from build123d import *

# Parameters (mm, degrees)
F1_W     = 100
F1_H     = 50
F2_DEPTH = 15
F3_R     = 10
F4_R     = 10
F5_W     = 40
F5_H     = 5
F6_DEPTH = 50.001
F7_T     = -3


with BuildPart() as f2:
    # F1 (on Front) → F2 (new body)
    with BuildSketch(Plane.XZ):
        with Locations((50, 25)):
            Rectangle(F1_W, F1_H)
    extrude(amount=F2_DEPTH)

    # F3
    f3_edges = [f2.edges().sort_by_distance(p)[0] for p in [
        (100, -7.5, 50),
    ]]
    fillet(f3_edges, radius=F3_R)

    # F4
    f4_edges = [f2.edges().sort_by_distance(p)[0] for p in [
        (100, -7.5, 0),
    ]]
    fillet(f4_edges, radius=F4_R)

    # F5 (on face) → F6 (cut, through all)
    with BuildSketch(Plane(origin=(0, 0, 0), x_dir=(1, 0, 0), z_dir=(0, 0, -1))):
        with Locations((50, 12.5)):
            Rectangle(F5_W, F5_H)
    extrude(amount=-F6_DEPTH, mode=Mode.SUBTRACT)

    # F7
    f7_openings = [f2.faces().sort_by_distance(p)[0] for p in [
        (49.58642, 0, 25),
    ]]
    offset(amount=F7_T, openings=f7_openings, kind=Kind.INTERSECTION)


solid = f2.part
Here's how the part is built. I have some questions about the finished solid (model axes, mm). A direction names the side the tool comes from. Round coordinates to 2 decimals unless told otherwise and drop trailing zeros. Loops run counter-clockwise (first coordinate to the right, second up) from the corner with the lowest first, then second, coordinate; pieces in that order, holes last. Notation, with made-up numbers: (-38.5, 79) -> (16.5, 79) arc R18 cw to (16.5, 83) -> close; hole circle Ø4 at (44, 59.25). An arc over 180 degrees is marked (long way). Write each question's results on one line, items separated by ' | '.
(1) For faces 5 (the face through (0, -7, 25)), 6 (the face through (50, -10, 25)), 7 (the face through (3, -6, 25)), which set-ups out of +Z, -Z, +X, -X, +Y, -Y let a thin tool reach every point of the face, with its end or its side?
Worked answers:
face 5: +Z, -Z, -X, +Y, -Y | face 6: +Z, -Z, -Y | face 7: +Y
(2) For P1, Ø2, axis at x = 79.5, z = 17, coming from the +Y side; P2, Ø2, axis at x = 61, z = 32.5, coming from the -Y side, each with a flat end and sliding along its axis, tell me the tip position at first contact or that it passes through.
Worked answers:
P1: y = -12 | P2: y = -10
(3) If I drill on L1, parallel to X at y = -8.75, z = 23.5; L2, parallel to Z at x = 9, y = -1.25; L3, parallel to X at y = -11.75, z = 9.5, over which ranges is the centre line in solid material (lowest first)?
Worked answers:
L1: 0 to 3, 27 to 73, 97 to 100 | L2: 0 to 3, 47 to 50 | L3: 0 to 3, 27 to 30, 70 to 73, 96.98 to 99.99
(4) If we section it at B-B, the plane x = 18: List the corners of the cut face in (y, z) for me.
Worked answers:
outline: (-15, 0) -> (0, 0) -> (0, 3) -> (-12, 3) -> (-12, 47) -> (0, 47) -> (0, 50) -> (-15, 50) -> close
(5) If we section it at C-C, the plane y = -9: List the corners of the cut face in (x, z) for me, then the cut area to 3 significant figures.
Worked answers:
outline: (0, 0) -> (90, 0) arc R10 ccw to (100, 10) -> (100, 40) arc R10 ccw to (90, 50) -> (0, 50) -> close; hole (3, 3) -> (27, 3) -> (27, 47) -> (3, 47) -> close; hole (73, 3) -> (90, 3) arc R7 ccw to (97, 10) -> (97, 40) arc R7 ccw to (90, 47) -> (73, 47) -> close | area: 2,870 mm2
(6) If we section it at D-D, the plane z = 22: List the corners of the cut face in (x, y) for me.
Worked answers:
outline: (0, -15) -> (30, -15) -> (30, -10) -> (70, -10) -> (70, -15) -> (100, -15) -> (100, 0) -> (97, 0) -> (97, -12) -> (73, -12) -> (73, -7) -> (27, -7) -> (27, -12) -> (3, -12) -> (3, 0) -> (0, 0) -> close
(7) We'd pull the mould along X, two halves only. Please class faces 1 (the face through (44, -6, 0)), 2 (the face through (50, -7, 25)), 3 (the face through (46, -5, 47)), 4 (the face through (97.15, -7.6, 46.99)): released by +X, released by -X, zero draft, split by the parting line, or undercut.
Worked answers:
face 1: zero draft | face 2: undercut | face 3: undercut | face 4: released by +X
(8) If we section it at A-A, the plane y = -4: List the corners of the cut face in (x, z) for me.
Worked answers:
outline: (0, 0) -> (90, 0) arc R10 ccw to (100, 10) -> (100, 40) arc R10 ccw to (90, 50) -> (0, 50) -> close; hole (3, 3) -> (90, 3) arc R7 ccw to (97, 10) -> (97, 40) arc R7 ccw to (90, 47) -> (3, 47) -> close
